from build123d import *

# Parameters (mm, degrees)
F0_W     = 812.8
F0_H     = 82.55
F1_DEPTH = 6.35
F3_DEPTH = 6.35
F5_DEPTH = 6.35


# Not quite as in the source:
# - a pattern or mirror of a feature is missing from the dataset's text; its kind, count and spacing are read off the source's solid


with BuildPart() as f1:
    # F0 (on Front) → F1 (new body)
    with BuildSketch(Plane.XZ):
        Rectangle(F0_W, F0_H)
    extrude(amount=F1_DEPTH)

    # F2 (on face) → F3 (cut, through all)
    with BuildSketch(Plane.XZ.offset(6.35)):
        with BuildLine():
            ThreePointArc((-254.508, 15.24), (-257.9768409794, 16.6768409794), (-256.54, 13.208))
            Line((-256.54, 13.208), (-256.54, 15.24))
            Line((-256.54, 15.24), (-254.508, 15.24))
        make_face()
        with BuildLine():
            Line((-256.54, 15.24), (-256.54, 13.208))
            ThreePointArc((-256.54, 13.208), (-255.1031590206, 13.8031590206), (-254.508, 15.24))
            Line((-254.508, 15.24), (-256.54, 15.24))
        make_face()
        with BuildLine():
            Line((-241.3, 0), (-255.5875, 0))
            ThreePointArc((-255.5875, 0), (-241.3, -14.2875), (-227.0125, 0))
            ThreePointArc((-227.0125, 0), (-231.1972118638, 10.1027881362), (-241.3, 14.2875))
            Line((-241.3, 14.2875), (-241.3, 0))
        make_face()
        with BuildLine():
            ThreePointArc((-241.3, 14.2875), (-251.4027881362, 10.1027881362), (-255.5875, 0))
            Line((-255.5875, 0), (-241.3, 0))
            Line((-241.3, 0), (-241.3, 14.2875))
        make_face()
        with BuildLine():
            Line((-256.54, -15.24), (-256.54, -13.208))
            ThreePointArc((-256.54, -13.208), (-257.9768409794, -16.6768409794), (-254.508, -15.24))
            Line((-254.508, -15.24), (-256.54, -15.24))
        make_face()
        with BuildLine():
            ThreePointArc((-254.508, -15.24), (-255.1031590206, -13.8031590206), (-256.54, -13.208))
            Line((-256.54, -13.208), (-256.54, -15.24))
            Line((-256.54, -15.24), (-254.508, -15.24))
        make_face()
        with BuildLine():
            Line((-226.06, -15.24), (-228.092, -15.24))
            ThreePointArc((-228.092, -15.24), (-226.06, -17.272), (-224.028, -15.24))
            ThreePointArc((-224.028, -15.24), (-224.6231590206, -13.8031590206), (-226.06, -13.208))
            Line((-226.06, -13.208), (-226.06, -15.24))
        make_face()
        with BuildLine():
            ThreePointArc((-226.06, -13.208), (-227.4968409794, -13.8031590206), (-228.092, -15.24))
            Line((-228.092, -15.24), (-226.06, -15.24))
            Line((-226.06, -15.24), (-226.06, -13.208))
        make_face()
        with BuildLine():
            ThreePointArc((-224.028, 15.24), (-227.4968409794, 16.6768409794), (-226.06, 13.208))
            ThreePointArc((-226.06, 13.208), (-224.6231590206, 13.8031590206), (-224.028, 15.24))
        make_face()
        with BuildLine():
            ThreePointArc((14.2875, 0), (10.1027881362, 10.1027881362), (0, 14.2875))
            ThreePointArc((0, 14.2875), (-10.1027881362, -10.1027881362), (14.2875, 0))
        make_face()
        with BuildLine():
            Line((15.24, -15.24), (13.208, -15.24))
            ThreePointArc((13.208, -15.24), (15.24, -17.272), (17.272, -15.24))
            ThreePointArc((17.272, -15.24), (16.6768409794, -13.8031590206), (15.24, -13.208))
            Line((15.24, -13.208), (15.24, -15.24))
        make_face()
        with BuildLine():
            ThreePointArc((15.24, -13.208), (13.8031590206, -13.8031590206), (13.208, -15.24))
            Line((13.208, -15.24), (15.24, -15.24))
            Line((15.24, -15.24), (15.24, -13.208))
        make_face()
        with BuildLine():
            ThreePointArc((17.272, 15.24), (13.8031590206, 16.6768409794), (15.24, 13.208))
            ThreePointArc((15.24, 13.208), (16.6768409794, 13.8031590206), (17.272, 15.24))
        make_face()
        with BuildLine():
            Line((-15.24, 15.24), (-13.208, 15.24))
            ThreePointArc((-13.208, 15.24), (-16.6768409794, 16.6768409794), (-15.24, 13.208))
            Line((-15.24, 13.208), (-15.24, 15.24))
        make_face()
        with BuildLine():
            ThreePointArc((-15.24, 13.208), (-13.8031590206, 13.8031590206), (-13.208, 15.24))
            Line((-13.208, 15.24), (-15.24, 15.24))
            Line((-15.24, 15.24), (-15.24, 13.208))
        make_face()
        with BuildLine():
            Line((-15.24, -15.24), (-15.24, -13.208))
            ThreePointArc((-15.24, -13.208), (-16.6768409794, -16.6768409794), (-13.208, -15.24))
            Line((-13.208, -15.24), (-15.24, -15.24))
        make_face()
        with BuildLine():
            ThreePointArc((-13.208, -15.24), (-13.8031590206, -13.8031590206), (-15.24, -13.208))
            Line((-15.24, -13.208), (-15.24, -15.24))
            Line((-15.24, -15.24), (-13.208, -15.24))
        make_face()
    f3 = extrude(amount=-F3_DEPTH, mode=Mode.SUBTRACT)

    # F3_copies: F3 across plane
    add(f3.mirror(Plane(origin=(120.65, 0, 0), x_dir=(0, 0, 1), z_dir=(1, 0, 0))), mode=Mode.SUBTRACT)

    # F4 (on face) → F5 (cut, through all)
    with BuildSketch(Plane.XZ.offset(6.35)):
        with BuildLine():
            ThreePointArc((-391.16, 26.035), (-391.9039487758, 27.8310512242), (-393.7, 28.575))
            Line((-393.7, 28.575), (-393.7, 23.495))
            ThreePointArc((-393.7, 23.495), (-391.9039487758, 24.2389487758), (-391.16, 26.035))
        make_face()
        with BuildLine():
            ThreePointArc((-391.16, -26.035), (-391.9039487758, -24.2389487758), (-393.7, -23.495))
            Line((-393.7, -23.495), (-393.7, -28.575))
            ThreePointArc((-393.7, -28.575), (-391.9039487758, -27.8310512242), (-391.16, -26.035))
        make_face()
        with BuildLine():
            Line((-393.7, -28.575), (-393.7, -23.495))
            ThreePointArc((-393.7, -23.495), (-396.24, -26.035), (-393.7, -28.575))
        make_face()
        with BuildLine():
            Line((-393.7, 23.495), (-393.7, 28.575))
            ThreePointArc((-393.7, 28.575), (-396.24, 26.035), (-393.7, 23.495))
        make_face()
        with BuildLine():
            ThreePointArc((-118.11, 26.035), (-118.8539487758, 27.8310512242), (-120.65, 28.575))
            Line((-120.65, 28.575), (-120.65, 23.495))
            ThreePointArc((-120.65, 23.495), (-118.8539487758, 24.2389487758), (-118.11, 26.035))
        make_face()
        with BuildLine():
            ThreePointArc((-118.11, -26.035), (-118.8539487758, -24.2389487758), (-120.65, -23.495))
            Line((-120.65, -23.495), (-120.65, -28.575))
            ThreePointArc((-120.65, -28.575), (-118.8539487758, -27.8310512242), (-118.11, -26.035))
        make_face()
        with BuildLine():
            Line((-120.65, -28.575), (-120.65, -23.495))
            ThreePointArc((-120.65, -23.495), (-123.19, -26.035), (-120.65, -28.575))
        make_face()
        with BuildLine():
            Line((-120.65, 23.495), (-120.65, 28.575))
            ThreePointArc((-120.65, 28.575), (-123.19, 26.035), (-120.65, 23.495))
        make_face()
    f5 = extrude(amount=-F5_DEPTH, mode=Mode.SUBTRACT)

    # F5_copies: F5 across plane
    add(f5.mirror(Plane(origin=(0, 0, 0), x_dir=(0, 0, 1), z_dir=(1, 0, 0))), mode=Mode.SUBTRACT)


solid = f1.part
Model file for the job. Use its own axes, mm. Coordinates: 2 decimals unless noted, no trailing zeros. Order: outer loops, then holes, each group sorted by start corner. A loop starts at its lowest first (then second) coordinate and runs counter-clockwise, first axis right, second up. Notation, with made-up numbers: M 18,52 L 33,52 A12 ccw 33,61 Z; hole C 19,61.25 d1. An arc over 180 degrees is marked long. Return JSON: item names as keys, results as strings.
1. Saw through at B-B (z = 0). Give the cut face in (x, y), and give its area (3 significant figures).
Ans:
{"outline": "M -406.4,-6.35 L -255.59,-6.35 L -255.59,0 L -406.4,0 Z; M -227.01,-6.35 L -14.29,-6.35 L -14.29,0 L -227.01,0 Z; M 14.29,-6.35 L 227.01,-6.35 L 227.01,0 L 14.29,0 Z; M 255.59,-6.35 L 406.4,-6.35 L 406.4,0 L 255.59,0 Z", "area": "4,620 mm^2"}
2. Pull direction X, two halves, no side cores. Call faces 1 (the face through (-227.352, -3.219, -3.097)), 2 (the face through (-6, -6.35, -18)): +X half, -X half, draft (parallel to the pull), parting line (faces both ways), or undercut.
Ans:
{"face 1": "undercut", "face 2": "draft"}
3. Saw through at C-C (y = -3.5). Give the number of separate pieces and of enclosed holes in the cut face, and give its area (3 significant figures).
Ans:
{"separate pieces": "1", "enclosed holes": "23", "area": "64,900 mm^2"}
4. Drill centre lines: probe 1 along Z at (x, y) = (-15.24, -4) (3 decimals); probe 2 along X at (y, z) = (-2, 0); probe 3 along X at (y, z) = (-4.25, -6). Where is each one in solid material? Low to high.
Ans:
{"probe 1": "-41.275 to -17.272, -13.208 to 13.208, 17.272 to 41.275", "probe 2": "-406.4 to -255.59, -227.01 to -14.29, 14.29 to 227.01, 255.59 to 406.4", "probe 3": "-406.4 to -254.27, -228.33 to -12.97, 12.97 to 228.33, 254.27 to 406.4"}
5. Flat gauge pins, fed straight in: pin 1 (5.5 mm diameter, centred on x = 256.54, z = 15.24, fed in from +Y); pin 2 (3.5 mm diameter, centred on x = -15.24, z = -15.24, fed in from -Y). Where does each tip first touch, or does it go through?
Ans:
{"pin 1": "y = 0", "pin 2": "through"}
